Verification items for the finished model (mm, model axes). Face numbers are marked on the shaded views. A direction names the side the tool comes from. Give positions to 0.01 mm unless a question says otherwise; leave off trailing zeros. Order: outer loops, then holes, each group sorted by start corner. A loop starts at its lowest first (then second) coordinate and runs counter-clockwise, first axis right, second up.
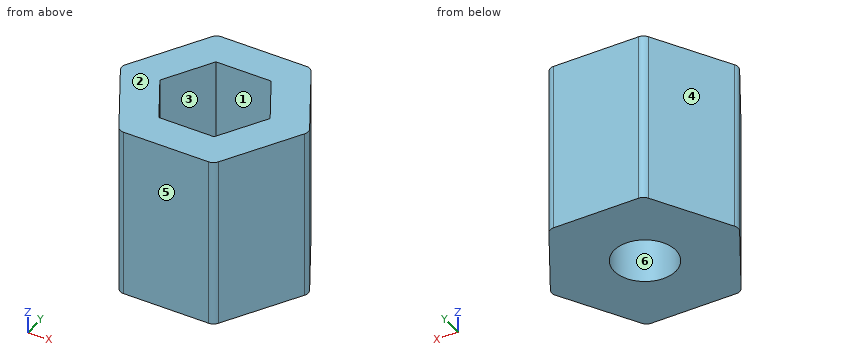
Autodesk Inventor part; units mm, degrees
ref_plane "YZ Plane" through (0, 0, 0) normal (1, 0, 0) x (0, 1, 0)
ref_plane "XZ Plane" through (0, 0, 0) normal (0, 1, 0) x (-1, 0, 0)
ref_plane "XY Plane" through (0, 0, 0) normal (0, 0, 1) x (1, 0, 0)
sketch "Sketch1" plane through (0, 0, 0) normal (0, 0, 1) x (1, 0, 0)
  circle A0 centre (0.0756, -0.4532) radius 1.5
  circle A1 centre (0.0756, -0.4532) radius 1.7
  circle A2 centre (0.0756, -0.4532) radius 1.7
  circle A3 centre (0.0756, -0.4532) radius 1.8
  line L0 (2.8469, 4.3468) -> (5.6182, -0.4532)
  line L1 (5.6182, -0.4532) -> (2.8469, -5.2532)
  line L2 (2.8469, -5.2532) -> (-2.6957, -5.2532)
  line L3 (-2.6957, -5.2532) -> (-5.4669, -0.4532)
  line L4 (-5.4669, -0.4532) -> (-2.6957, 4.3468)
  line L5 (-2.6957, 4.3468) -> (2.8469, 4.3468)
  line L6 (-1.558, 1.3468) -> (2.6621, 1.3468) construction
  point P0 (0, 0)
  dimension "d0" = 0.1
  dimension "d1" = 3
extrude "Extrusion1" add sketch "Sketch1" along normal blind 4 contours L0 L1 L2 L3 L4 L5
sketch "Sketch2" plane through (0, 0, 4) normal (0, 0, 1) x (1, 0, 0)
  line L0 (-2.6957, 4.3468) -> (-5.4669, -0.4532)
  line L1 (-5.4669, -0.4532) -> (-2.6957, -5.2532)
  line L2 (-2.6957, -5.2532) -> (2.8469, -5.2532)
  line L3 (2.8469, -5.2532) -> (5.6182, -0.4532)
  line L4 (5.6182, -0.4532) -> (2.8469, 4.3468)
  line L5 (2.8469, 4.3468) -> (-2.6957, 4.3468)
  circle A0 centre (0.0756, -0.4532) radius 1.8
  line L6 (-3.1575, -0.4532) -> (-1.541, 2.3468)
  line L7 (-1.541, 2.3468) -> (1.6922, 2.3468)
  line L8 (1.6922, 2.3468) -> (3.3088, -0.4532)
  line L9 (3.3088, -0.4532) -> (1.6922, -3.2532)
  line L10 (1.6922, -3.2532) -> (-1.541, -3.2532)
  line L11 (-1.541, -3.2532) -> (-3.1575, -0.4532)
  point P0 (0, 0)
  dimension "d4" = 2
extrude "Extrusion2" add sketch "Sketch2" along normal blind 6 contours L5 L4 L3 L2 L1 L0
fillet "Fillet1" radius 0.5 6 edges at (-5.4669, -0.4532, 5) (-2.6957, 4.3468, 5) (2.8469, 4.3468, 5) (5.6182, -0.4532, 5) (-2.6957, -5.2532, 5) (2.8469, -5.2532, 5)
thread "Thread1"
properties part number "TurretTighteningNut"
(1) Go/stop test with flat-tipped pins: pin 1 (1 mm diameter, centred on y = 2, z = 6.5, fed in from +X); pin 2 (4 mm diameter, centred on x = 0, y = -0.5, fed in from +Z); pin 3 (1.5 mm diameter, centred on y = -3, z = 1, fed in from +X). Record where each tip stops, or that it passes through.
Solved:
pin 1: stops at x = 4.49
pin 2: stops at z = 4
pin 3: stops at x = 4.58
(2) Section check D-D, the plane x = 2.75. Enter the section's corners in (y, z).
Solved:
outline: (-5.21, 0) - (4.31, 0) - (4.31, 10) - (0.51, 10) - (0.51, 4) - (-1.42, 4) - (-1.42, 10) - (-5.21, 10) - close
(3) Release check for a two-part mould opening along Y. For the marked faces 3, 4, 5 and 6 record: pulls with the +Y half, pulls with the -Y half, needs draft (parallel to the pull), parting line crosses it, or undercut.
Solved:
face 3: undercut
face 4: pulls with the +Y half
face 5: pulls with the -Y half
face 6: undercut
(4) Section check A-A, the plane y = -1. Enter the section's corners in (x, z).
Solved:
outline: (-5.15, 0) - (-1.64, 0) - (-1.64, 4) - (-2.84, 4) - (-2.84, 10) - (-5.15, 10) - close; (1.79, 0) - (5.3, 0) - (5.3, 10) - (2.99, 10) - (2.99, 4) - (1.79, 4) - close
(5) Set-up check for the marked faces 1 and 2: record each of +Z, -Z, +X, -X, +Y, -Y from which the full face is reachable in a straight line by a thin tool's end or side.
Solved:
face 1: +Z
face 2: +Z, +X, -X, +Y, -Y
(6) Scan lines: line 1 (Y direction, x = 0.5, z = 7.25); line 2 (Y direction, x = 4, z = 3.5); line 3 (Y direction, x = -1.5, z = 2.25). Record each from-to range of solid material in increasing order.
Solved:
line 1: y = -5.25 to -3.25, 2.35 to 4.35
line 2: y = -3.26 to 2.35
line 3: y = -5.25 to -1.32, 0.42 to 4.35
(7) Section check B-B, the plane z = 4.25. Enter the section's corners in (x, y).
Solved:
outline: (-5.32, -0.7) - (-2.84, -5) arc R0.5 ccw to (-2.41, -5.25) - (2.56, -5.25) arc R0.5 ccw to (2.99, -5) - (5.47, -0.7) arc R0.5 ccw to (5.47, -0.2) - (2.99, 4.1) arc R0.5 ccw to (2.56, 4.35) - (-2.41, 4.35) arc R0.5 ccw to (-2.84, 4.1) - (-5.32, -0.2) arc R0.5 ccw to start; hole (-3.16, -0.45) - (-1.54, -3.25) - (1.69, -3.25) - (3.31, -0.45) - (1.69, 2.35) - (-1.54, 2.35) - close
(8) Section check C-C, the plane x = 0.5. Enter the section's corners in (y, z).
Solved:
outline: (-5.25, 0) - (-2.2, 0) - (-2.2, 4) - (-3.25, 4) - (-3.25, 10) - (-5.25, 10) - close; (1.3, 0) - (4.35, 0) - (4.35, 10) - (2.35, 10) - (2.35, 4) - (1.3, 4) - close
